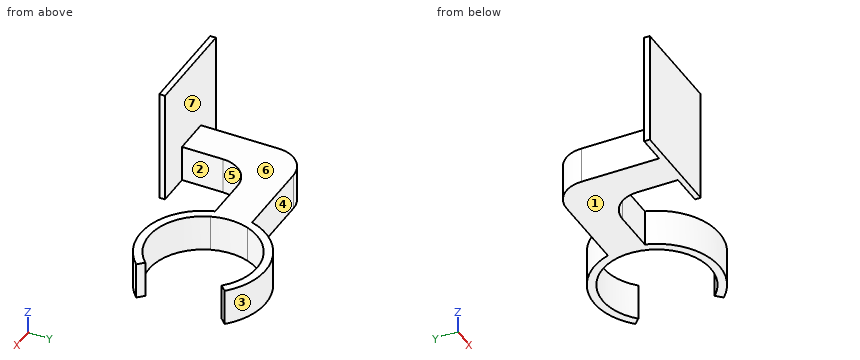
from build123d import *

# Parameters (mm, degrees)
F0_W     = 13
F0_H     = 25
F1_DEPTH = 12.8
F2_DEPTH = 40
F3_R     = 10.6225396744


with BuildPart() as f1:
    # F0 (on Top) → F1 (new body)
    with BuildSketch(Plane.XY):
        with BuildLine():
            ThreePointArc((-21.017849557, -6.5), (-22, 0), (-21.017849557, 6.5))
            Line((-21.017849557, 6.5), (-60, 6.5))
            Line((-60, 6.5), (-60, -6.5))
            Line((-60, -6.5), (-47, -6.5))
            Line((-47, -6.5), (-21.017849557, -6.5))
        make_face()
        with Locations((-53.5, -19)):
            Rectangle(F0_W, F0_H)
        with BuildLine():
            ThreePointArc((-17.8535710714, -6.5), (-19, 0), (-17.8535710714, 6.5))
            Line((-17.8535710714, 6.5), (-21.017849557, 6.5))
            ThreePointArc((-21.017849557, 6.5), (-22, 0), (-21.017849557, -6.5))
            Line((-21.017849557, -6.5), (-17.8535710714, -6.5))
        make_face()
        with BuildLine():
            Line((15.5563491861, -15.5563491861), (13.4350288425, -13.4350288425))
            ThreePointArc((13.4350288425, -13.4350288425), (-4.1115125099, -18.5498103732), (-17.8535710714, -6.5))
            Line((-17.8535710714, -6.5), (-21.017849557, -6.5))
            ThreePointArc((-21.017849557, -6.5), (-5.2878503875, -21.3550611865), (15.5563491861, -15.5563491861))
        make_face()
        with BuildLine():
            ThreePointArc((-17.8535710714, 6.5), (-4.1115125099, 18.5498103732), (13.4350288425, 13.4350288425))
            Line((13.4350288425, 13.4350288425), (15.5563491861, 15.5563491861))
            ThreePointArc((15.5563491861, 15.5563491861), (-5.2878503875, 21.3550611865), (-21.017849557, 6.5))
            Line((-21.017849557, 6.5), (-17.8535710714, 6.5))
        make_face()
    extrude(amount=F1_DEPTH)

    # F0 (on Top) → F2 (join)
    with BuildSketch(Plane.XY):
        Polygon((-35.3286863863, -31.5), (-47, -31.5), (-60, -31.5), (-70.3286863863, -31.5), (-70.3286863863, -33.5), (-35.3286863863, -33.5), align=None)
    extrude(amount=F2_DEPTH)

    # F3
    f3_edges = [f1.edges().sort_by_distance(p)[0] for p in [
        (-60, 6.5, 6.4),
        (-47, -6.5, 6.4),
    ]]
    fillet(f3_edges, radius=F3_R)


solid = f1.part
The listing builds one solid part. Answer for the finished solid, in the listing's coordinates (mm). Face numbers are marked on the shaded views. A direction names the side the tool comes from. Round coordinates to 2 decimals unless told otherwise and drop trailing zeros. Write each loop counter-clockwise with the first axis right and the second up, starting at its lowest first coordinate (ties: lowest second). Pieces come first, ordered by that corner, then holes. Notation, with made-up numbers: M 25,21 L 54,21 A22 cw 54,57 Z; hole C 14,28.5 d7. An arc over 180 degrees is marked long. Write each question's results on one line, items separated by ' | '. Start each with the question number.
(1) Each of these flat-tipped pins is pushed along its axis until it touches: P1, Ø14, axis at x = -41.5, z = 6, coming from the +Y side; P2, Ø6.5, axis at y = -18.5, z = 9, coming from the -X side; P3, Ø16, axis at x = -22.5, y = -12, coming from the +Z side. Where does it stop, or does it pass through?
(2) The part is cut by section A-A, the plane x = -44. Write down the section's boundary in (y, z), and give its area (3 significant figures).
(3) Find the intervals of material crossed by line 1 (Y direction, x = -44.5, z = 15); line 2 (Z direction, x = -32.5, y = 2.5); line 3 (X direction, y = 17.5, z = 7.5), in increasing order.
(4) Determine the mould class of the marked faces 1, 2 and 3 for opening direction Y: +Y half, -Y half, draft (parallel to the pull), parting line (faces both ways), or undercut.
(5) The part is cut by section B-B, the plane z = 8. Write down the section's boundary in (x, y).
(6) The part is cut by section C-C, the plane y = -12. Write down the section's boundary in (x, z), and give its area (3 significant figures).
(7) The part is cut by section D-D, the plane y = -27. Write down the section's boundary in (x, z), and give its area (3 significant figures).
(8) For the marked faces 4, 5, 6 and 7, determine the directions among +Z, -Z, +X, -X, +Y, -Y from which every point of the face is accessible in a straight line to the end or side of a thin tool.
Worked answers:
1) P1: stops at y = 6.5 | P2: stops at x = -60 | P3: stops at z = 12.8
2) outline: M -33.5,0 L -31.5,0 L -31.5,40 L -33.5,40 Z; M -9.72,0 L 6.5,0 L 6.5,12.8 L -9.72,12.8 Z | area: 288 mm²
3) line 1: y = -33.5 to -31.5 | line 2: z = 0 to 12.8 | line 3: x = -13.33 to -7.4, 7.4 to 13.33
4) face 1: draft | face 2: undercut | face 3: +Y half
5) outline: M -70.33,-33.5 L -35.33,-33.5 L -35.33,-31.5 L -47,-31.5 L -47,-17.12 A10.62 cw -36.38,-6.5 L -21.02,-6.5 A22 ccw 15.56,-15.56 L 13.44,-13.44 A19 cw long 13.44,13.44 L 15.56,15.56 A22 ccw -21.02,6.5 L -49.38,6.5 A10.62 ccw -60,-4.12 L -60,-31.5 L -70.33,-31.5 Z
6) outline: M -60,0 L -45.68,0 L -45.68,12.8 L -60,12.8 Z; M -18.44,0 L -14.73,0 L -14.73,12.8 L -18.44,12.8 Z | area: 231 mm²
7) outline: M -60,0 L -47,0 L -47,12.8 L -60,12.8 Z | area: 166 mm²
8) face 4: +Z, -Z, -X, +Y | face 5: +Z, -Z | face 6: +Z, +X, -X, +Y | face 7: +Z
